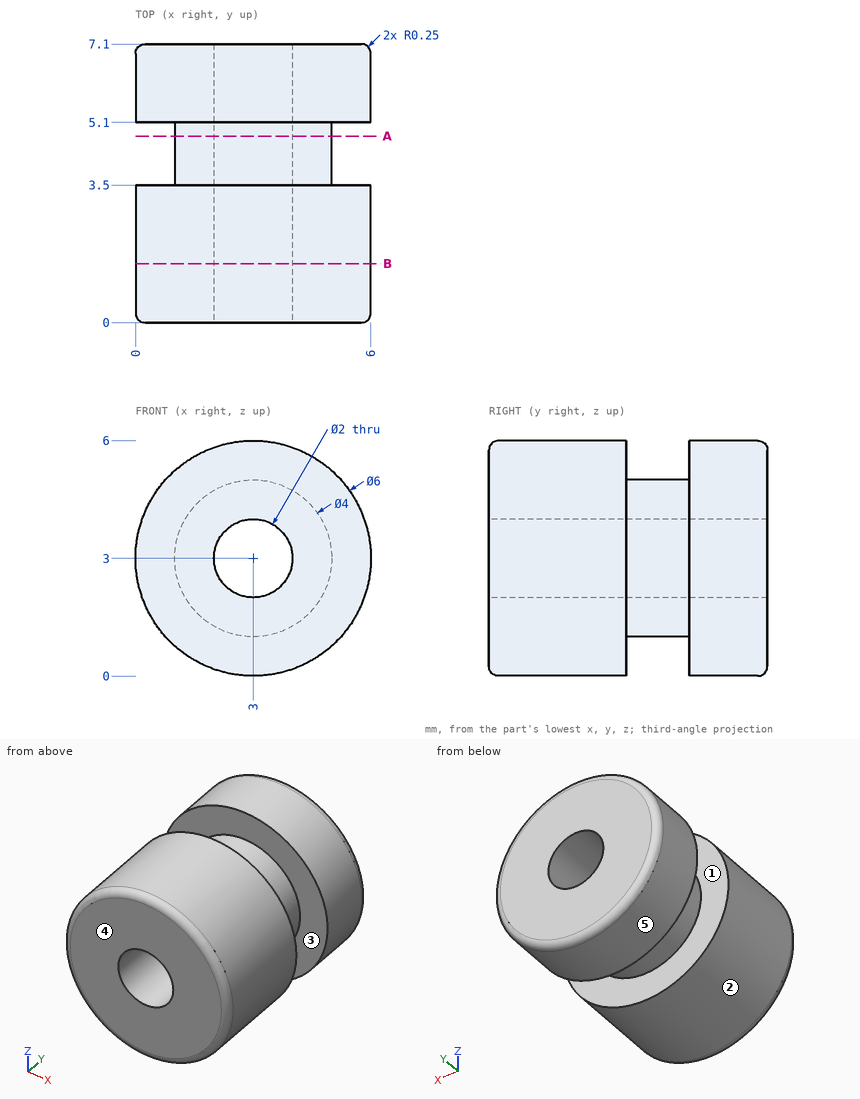
Geometry: see drawing. Coordinates: mm, zero at the bounding-box minimum. A direction names the side the tool comes from. Round coordinates to 2 decimals unless told otherwise and drop trailing zeros. Loops run counter-clockwise (first coordinate to the right, second up) from the corner with the lowest first, then second, coordinate; pieces in that order, holes last. Notation, with made-up numbers: (-0.5, 78.25) -> (51.5, 78.25) arc R11 ccw to (51.5, 84.25) -> close; hole circle Ø3 at (50.5, 10.5). An arc over 180 degrees is marked (long way). One line per question, with ' | ' between items. Start each with the question number.
1. Contact query for flat-ended pins moving along their axis: pin 1 (1.6 mm diameter, centred on x = 3, z = 3, fed in from -Y); pin 2 (2 mm diameter, centred on y = 2, z = 5, fed in from +X); pin 3 (1 mm diameter, centred on x = 5, y = 6, fed in from -Z); pin 4 (3 mm diameter, centred on x = 2.5, z = 3, fed in from +Y). Output: stop coordinate, or through.
2. Section B-B on y = 1.5. Output: boundary loops of the cut face in (x, z), and give its area (3 significant figures).
3. Set-up query: the marked faces 1 and 2. Return all of +Z, -Z, +X, -X, +Y, -Y with unobstructed straight access to the full face (end or side cutting, diameter ignored); none if empty.
4. Mould query, pull axis Y, two halves, no side actions, for the marked faces 3, 4 and 5. Classes: pulls with the +Y half, pulls with the -Y half, needs draft (parallel to the pull), parting line crosses it, or undercut.
5. Section A-A on y = 4.75. Output: boundary loops of the cut face in (x, z), and give its area (3 significant figures).
6. Line query: line 1 along Y through (x, z) = (4.25, 5); line 2 along Z through (x, y) = (3, 2.75); line 3 along Z through (x, y) = (3, 5). Output: solid intervals per line, ascending. Write a range as [from, to].
Returned:
1) pin 1: passes through | pin 2: stops at x = 5.83 | pin 3: stops at z = 0.4 | pin 4: stops at y = 7.1
2) outline: circle Ø6 at (3, 3); hole circle Ø2 at (3, 3) | area: 25.1 mm2
3) face 1: none | face 2: +Y, -Y
4) face 3: undercut | face 4: pulls with the -Y half | face 5: needs draft
5) outline: circle Ø4 at (3, 3); hole circle Ø2 at (3, 3) | area: 9.42 mm2
6) line 1: y = [0, 3.5], [5.1, 7.1] | line 2: z = [0, 2], [4, 6] | line 3: z = [1, 2], [4, 5]
